Check sheet for the modelled part. Datum: model origin and axes. Units: mm. A direction names the side the tool comes from. Coordinates: 2 decimals unless noted, no trailing zeros. One line per item, written item: value. Start each with the question number.
1) Sectioned sample at A-A on z = 313.5. Give the number of separate pieces and of enclosed holes in the cut face, plus the area to 3 significant figures.
2) Scan lines: line 1 along X through (y, z) = (-9.75, 290); line 2 along Y through (x, z) = (-25, 271); line 3 along Y through (x, z) = (15, 262.5). Record each from-to range of solid material in increasing order. Write a range as [from, to].
3) Draft check along X on faces 3 (the flat face through (0, -12.5, 168)), 4 (the flat face through (30, 9, 168)), 5 (the flat face through (24, 15, 168)). Enter one of: +X half, -X half, draft (parallel to the pull), parting line (faces both ways), or undercut.
4) Set-up check for faces 1 (the flat face through (-7, -10, 168)), 2 (the flat face through (24, -15, 168)): record each of +Z, -Z, +X, -X, +Y, -Y from which the full face is reachable in a straight line by a thin tool's end or side.
```python
from build123d import *

# Parameters (mm, degrees)
F0_R     = 3
F0_R_2   = 2.5
F1_DEPTH = 340
F2_R     = 2
F3_R     = 7


# Not quite as in the source:
# - a feature names something its author has since deleted; it is built from what else it names


with BuildPart() as f1:
    # F0 (on Top) → F1 (new body)
    with BuildSketch(Plane.XY):
        with BuildLine():
            Line((18.15, -15), (30, -15))
            Line((30, -15), (30, -3.15))
            Line((30, -3.15), (27.5, -3.15))
            Line((27.5, -3.15), (27.5, -5.15))
            Line((27.5, -5.15), (21.5477069044, -5.15))
            ThreePointArc((21.5477069044, -5.15), (19.5, 0), (21.5477069044, 5.15))
            Line((21.5477069044, 5.15), (27.5, 5.15))
            Line((27.5, 5.15), (27.5, 3.15))
            Line((27.5, 3.15), (30, 3.15))
            Line((30, 3.15), (30, 15))
            Line((30, 15), (18.15, 15))
            Line((18.15, 15), (18.15, 12.5))
            Line((18.15, 12.5), (20.15, 12.5))
            Line((20.15, 12.5), (20.15, 6.5477069044))
            ThreePointArc((20.15, 6.5477069044), (15, 4.5), (9.85, 6.5477069044))
            Line((9.85, 6.5477069044), (9.85, 12.5))
            Line((9.85, 12.5), (11.85, 12.5))
            Line((11.85, 12.5), (11.85, 15))
            Line((11.85, 15), (-11.85, 15))
            Line((-11.85, 15), (-11.85, 12.5))
            Line((-11.85, 12.5), (-9.85, 12.5))
            Line((-9.85, 12.5), (-9.85, 6.5477069044))
            ThreePointArc((-9.85, 6.5477069044), (-15, 4.5), (-20.15, 6.5477069044))
            Line((-20.15, 6.5477069044), (-20.15, 12.5))
            Line((-20.15, 12.5), (-18.15, 12.5))
            Line((-18.15, 12.5), (-18.15, 15))
            Line((-18.15, 15), (-30, 15))
            Line((-30, 15), (-30, 3.15))
            Line((-30, 3.15), (-27.5, 3.15))
            Line((-27.5, 3.15), (-27.5, 5.15))
            Line((-27.5, 5.15), (-21.5477069044, 5.15))
            ThreePointArc((-21.5477069044, 5.15), (-19.5, 0), (-21.5477069044, -5.15))
            Line((-21.5477069044, -5.15), (-27.5, -5.15))
            Line((-27.5, -5.15), (-27.5, -3.15))
            Line((-27.5, -3.15), (-30, -3.15))
            Line((-30, -3.15), (-30, -15))
            Line((-30, -15), (-18.15, -15))
            Line((-18.15, -15), (-18.15, -12.5))
            Line((-18.15, -12.5), (-20.15, -12.5))
            Line((-20.15, -12.5), (-20.15, -6.5477069044))
            ThreePointArc((-20.15, -6.5477069044), (-15, -4.5), (-9.85, -6.5477069044))
            Line((-9.85, -6.5477069044), (-9.85, -12.5))
            Line((-9.85, -12.5), (-11.85, -12.5))
            Line((-11.85, -12.5), (-11.85, -15))
            Line((-11.85, -15), (11.85, -15))
            Line((11.85, -15), (11.85, -12.5))
            Line((11.85, -12.5), (9.85, -12.5))
            Line((9.85, -12.5), (9.85, -6.5477069044))
            ThreePointArc((9.85, -6.5477069044), (15, -4.5), (20.15, -6.5477069044))
            Line((20.15, -6.5477069044), (20.15, -12.5))
            Line((20.15, -12.5), (18.15, -12.5))
            Line((18.15, -12.5), (18.15, -15))
        make_face()
        with Locations((-25, -10)):
            Circle(F0_R, mode=Mode.SUBTRACT)
        with Locations((25, -10)):
            Circle(F0_R, mode=Mode.SUBTRACT)
        with Locations((-15, 0)):
            Circle(F0_R_2, mode=Mode.SUBTRACT)
        with Locations((-25, 10)):
            Circle(F0_R, mode=Mode.SUBTRACT)
        Polygon((-7, 7), (-7, 12.5), (0, 12.5), (7, 12.5), (7, 7), (10, 0), (7, -7), (7, -12.5), (0, -12.5), (-7, -12.5), (-7, -7), (-10, 0), align=None, mode=Mode.SUBTRACT)
        with Locations((15, 0)):
            Circle(F0_R_2, mode=Mode.SUBTRACT)
        with Locations((25, 10)):
            Circle(F0_R, mode=Mode.SUBTRACT)
    extrude(amount=F1_DEPTH)

    # F2
    f2_edges = [f1.edges().sort_by_distance(p)[0] for p in [
        (-7, 12.5, 170),
        (7, 12.5, 170),
    ]]
    fillet(f2_edges, radius=F2_R)

    # F3
    f3_edges = [f1.edges().sort_by_distance(p)[0] for p in [
        (-7, 7, 170),
        (-10, 0, 170),
        (7, 7, 170),
        (10, 0, 170),
    ]]
    fillet(f3_edges, radius=F3_R)


solid = f1.part
```
Answers:
1. separate pieces: 1
1. enclosed holes: 7
1. area: 710 mm2
2. line 1: x = [-30, -27.99], [-22.01, -20.15], [-9.85, -7], [7, 9.85], [20.15, 22.01], [27.99, 30]
2. line 2: y = [-15, -13], [-7, -5.15], [5.15, 7], [13, 15]
2. line 3: y = [-4.5, -2.5], [2.5, 4.5]
3. face 3: undercut
3. face 4: +X half
3. face 5: draft
4. face 1: +Z, -Z
4. face 2: +Z, -Z, +X, -X, -Y
